Build history of the part. All positions in model axes, mm. A direction names the side the tool comes from. Round coordinates to 2 decimals unless told otherwise and drop trailing zeros. Write each loop counter-clockwise with the first axis right and the second up, starting at its lowest first coordinate (ties: lowest second). Pieces come first, ordered by that corner, then holes. Notation, with made-up numbers: (32.25, -16.5) -> (87.25, -16.5) arc R29 ccw to (87.25, 5.5) -> close; hole circle Ø5 at (7.5, 72). An arc over 180 degrees is marked (long way). Answer in a Markdown table with one row per item.
```python
from build123d import *

# Parameters (mm, degrees)
BOSS_EXTRUDE1_DEPTH = 10
CHAMFER1_SIZE       = 10
CUT_EXTRUDE3_DEPTH  = 7
SKETCH7_R           = 4
CUT_EXTRUDE4_DEPTH  = 11
SKETCH8_R           = 1.5
CUT_EXTRUDE5_DEPTH  = 11
SKETCH9_W           = 50
SKETCH9_H           = 20
BOSS_EXTRUDE2_DEPTH = 20
CHAMFER2_SIZE       = 10
CHAMFER3_SIZE       = 5
SKETCH10_R          = 1.25
CUT_EXTRUDE6_DEPTH  = 10
CHAMFER4_SIZE       = 0.5


with BuildPart() as part:
    # Sketch1 → Boss-Extrude1 (new, symmetric)
    with BuildSketch(Plane.XY):
        with BuildLine():
            Line((25, 50), (25, 0))
            ThreePointArc((25, 0), (0, -25), (-25, 0))
            Line((-25, 0), (-25, 50))
            Line((-25, 50), (25, 50))
        make_face()
    extrude(amount=BOSS_EXTRUDE1_DEPTH, both=True)

    # Chamfer1
    chamfer1_edges = [part.edges().sort_by_distance(p)[0] for p in [
        (25, 25, -10),
        (0, -25, -10),
        (-25, 25, -10),
    ]]
    chamfer(chamfer1_edges, length=CHAMFER1_SIZE)

    # Sketch6 → Cut-Extrude3 (cut)
    with BuildSketch(Plane.XY.offset(10)):
        with BuildLine():
            Line((3.075, 10.981803131), (3.075, 24.5))
            ThreePointArc((3.075, 24.5), (-0.339576943, 27.556192484), (-3, 23.825))
            Line((-3, 23.825), (-3, 11.070484407))
            ThreePointArc((-3, 11.070484407), (-3.615579404, 7.616117595), (-5.386530015, 4.587038195))
            ThreePointArc((-5.386530015, 4.587038195), (-0.02406199, -7.074959083), (5.417606149, 4.550293244))
            ThreePointArc((5.417606149, 4.550293244), (3.678885417, 7.559372599), (3.075, 10.981803131))
        make_face()
    extrude(amount=-CUT_EXTRUDE3_DEPTH, mode=Mode.SUBTRACT)

    # Sketch7 → Cut-Extrude4 (cut)
    with BuildSketch(Plane(origin=(0, 0, -10), x_dir=(-1, 0, 0), z_dir=(0, 0, -1))):
        Circle(SKETCH7_R)
        with Locations((0, 24.5)):
            Circle(SKETCH7_R)
    extrude(amount=-CUT_EXTRUDE4_DEPTH, mode=Mode.SUBTRACT)

    # Sketch8 → Cut-Extrude5 (cut)
    with BuildSketch(Plane(origin=(0, 0, 1), x_dir=(-1, 0, 0), z_dir=(0, 0, -1))):
        with Locations((0, 24.5)):
            Circle(SKETCH8_R)
        Circle(SKETCH8_R)
    extrude(amount=-CUT_EXTRUDE5_DEPTH, mode=Mode.SUBTRACT)

    # Sketch9 → Boss-Extrude2 (add)
    with BuildSketch(Plane.XY.offset(10)):
        with Locations((0, 40)):
            Rectangle(SKETCH9_W, SKETCH9_H)
    extrude(amount=BOSS_EXTRUDE2_DEPTH)

    # Chamfer2
    chamfer2_edges = [part.edges().sort_by_distance(p)[0] for p in [
        (25, 30, 20),
        (-25, 30, 20),
        (25, 40, 30),
        (-25, 40, 30),
    ]]
    chamfer(chamfer2_edges, length=CHAMFER2_SIZE)

    # Chamfer3
    chamfer3_edges = [part.edges().sort_by_distance(p)[0] for p in [
        (-25, 50, 10),
        (25, 50, 10),
    ]]
    chamfer(chamfer3_edges, length=CHAMFER3_SIZE)

    # Sketch10 → Cut-Extrude6 (cut)
    with BuildSketch(Plane(origin=(0, 50, 0), x_dir=(1, 0, 0), z_dir=(0, 1, 0))):
        with Locations(Location((10, 5, 0), (0, 0, 270))):
            Circle(SKETCH10_R)
        with Locations(Location((10, -25, 0), (0, 0, 90))):
            Circle(SKETCH10_R)
        with Locations(Location((-10, -25, 0), (0, 0, 270))):
            Circle(SKETCH10_R)
        with Locations(Location((-10, 5, 0), (0, 0, 90))):
            Circle(SKETCH10_R)
    extrude(amount=-CUT_EXTRUDE6_DEPTH, mode=Mode.SUBTRACT)

    # Chamfer4
    chamfer4_edges = [part.edges().sort_by_distance(p)[0] for p in [
        (-10, 50, -3.75),
        (-10, 50, 23.75),
        (10, 50, 26.25),
        (10, 50, -6.25),
    ]]
    chamfer(chamfer4_edges, length=CHAMFER4_SIZE)


solid = part.part
```
Q1. Saw through at B-B on x = 0. Write the cut outline in (y, z) (3 decimals).
A:
| item | result |
|---|---|
| outline | (-25, 0) -> (-15, -10) -> (-4, -10) -> (-4, 1) -> (-1.5, 1) -> (-1.5, 3) -> (-7.075, 3) -> (-7.075, 10) -> (-25, 10) -> close; (1.5, 1) -> (4, 1) -> (4, -10) -> (20.5, -10) -> (20.5, 1) -> (23, 1) -> (23, 3) -> (1.5, 3) -> close; (26, 1) -> (28.5, 1) -> (28.5, -10) -> (50, -10) -> (50, 30) -> (30, 30) -> (30, 10) -> (27.575, 10) -> (27.575, 3) -> (26, 3) -> close |
Q2. Saw through at A-A on z = -1.5. Write the cut outline in (x, y).
A:
| item | result |
|---|---|
| outline | (-23.5, 0) arc R23.5 ccw to (23.5, 0) -> (23.5, 46.5) -> (20, 50) -> (-20, 50) -> (-23.5, 46.5) -> close; hole circle Ø8 at (0, 0); hole circle Ø8 at (0, 24.5) |
Q3. Two-plate mould, pull along X, no slides. Class faces 1 (the flat face through (-20, 25, -5)), 2 (the cylindrical face through (-11.24, 44.82, -4.84)), 3 (the cylindrical face through (0.55, -24.994, 5.07)): released by +X, released by -X, zero draft, split by the parting line, or undercut.
A:
| item | result |
|---|---|
| face 1 | released by -X |
| face 2 | undercut |
| face 3 | split by the parting line |
Q4. Saw through at C-C on y = 9.5. Write the cut outline in (x, z).
A:
| item | result |
|---|---|
| outline | (-25, 0) -> (-15, -10) -> (15, -10) -> (25, 0) -> (25, 10) -> (3.19, 10) -> (3.19, 3) -> (-3.12, 3) -> (-3.12, 10) -> (-25, 10) -> close |
Q5. Saw through at D-D on z = 14.5. Write the cut outline in (x, y).
A:
| item | result |
|---|---|
| outline | (-25, 40) -> (-15, 30) -> (15, 30) -> (25, 40) -> (25, 45) -> (20, 50) -> (-20, 50) -> (-25, 45) -> close |
Q6. Which spindle directions (+Z, -Z, +X, -X, +Y, -Y) get a long thin tool onto all of the face, cutting with end or side? Do faces 4 (the cylindrical face through (0, 26, 2)), 5 (the cylindrical face through (0.521, 28.466, -4.577)), 6 (the flat face through (10, 40, 25)), 7 (the cylindrical face through (-0.268, 27.563, 6.549)). Say none if no direction does.
A:
| item | result |
|---|---|
| face 4 | +Z, -Z |
| face 5 | -Z |
| face 6 | +Y |
| face 7 | +Z |
Q7. Wall check: line 1 (Y direction, x = 0, z = 8) (3 decimals); line 2 (Z direction, x = 5, y = 13); line 3 (Y direction, x = 0, z = -3.5). Give the ranges that are in metal, low to high. Write a range as [from, to].
A:
| item | result |
|---|---|
| line 1 | [-25, -7.075], [27.575, 50] |
| line 2 | [-10, 10] |
| line 3 | [-21.5, -4], [4, 20.5], [28.5, 50] |
Q8. Drop flat-ended pins along their axis: P1, Ø4, axis at x = -1, y = 1.5, coming from the -Z side; P2, Ø1, axis at x = 17, y = 32, coming from the -Z side; P3, Ø6.5, axis at x = 0, y = 24.5, coming from the +Z side; P4, Ø6, axis at y = 19.5, z = 11, coming from the -X side. Give the stop position or say it passes through.
A:
| item | result |
|---|---|
| P1 | z = 1 |
| P2 | z = -8.5 |
| P3 | z = 10 |
| P4 | x = -25 |
